Part model, mm, in its own coordinate system. A direction names the side the tool comes from. Coordinates: 2 decimals unless noted, no trailing zeros. Write each loop counter-clockwise with the first axis right and the second up, starting at its lowest first coordinate (ties: lowest second). Pieces come first, ordered by that corner, then holes. Notation, with made-up numbers: (-15, 59.5) - (-4, 59.5) arc R29 cw to (-4, 83.5) - close; hole circle Ø10 at (35, -10.75). An arc over 180 degrees is marked (long way). Use one line per item in the form item = value. Start each with the question number.
from build123d import *

# Parameters (mm, degrees)
SKETCH_1_W          = 367
SKETCH_1_H          = 337
EXTRUDE_1_DEPTH     = 200
SKETCH_2_W          = 245
SKETCH_2_H          = 47
EXTRUDE_2_DEPTH     = 47
SKETCH_3_W          = 18.503948035
SKETCH_3_H          = 22.759447516
EXTRUDE_3_DEPTH     = 35
SKETCH_4_R          = 4.689122638
EXTRUDE_4_DEPTH     = 70
CUT_EXTRUDE_1_DEPTH = 25
CUT_EXTRUDE_2_DEPTH = 223


with BuildPart() as part:
    # Эскиз1 → Бобышка-Вытянуть1 (new body)
    with BuildSketch(Plane(origin=(0, 0, 0), x_dir=(1, 0, 0), z_dir=(0, 1, 0))):
        with Locations((-16.254231815, -121.394753304)):
            Rectangle(SKETCH_1_W, SKETCH_1_H)
    extrude(amount=EXTRUDE_1_DEPTH)

    # Эскиз2 → Бобышка-Вытянуть2 (add)
    with BuildSketch(Plane(origin=(0, 0, -47.105246696), x_dir=(-1, 0, 0), z_dir=(0, 0, -1))):
        with Locations((16.254231815, 23.5)):
            Rectangle(SKETCH_2_W, SKETCH_2_H)
    extrude(amount=EXTRUDE_2_DEPTH)

    # Эскиз3 → Бобышка-Вытянуть3 (add)
    with BuildSketch(Plane(origin=(0, 0, -47.105246696), x_dir=(-1, 0, 0), z_dir=(0, 0, -1))):
        with Locations((-137.993794167, 26.379723758)):
            Rectangle(SKETCH_3_W, SKETCH_3_H)
    extrude(amount=EXTRUDE_3_DEPTH)

    # Эскиз4 → Бобышка-Вытянуть4 (add)
    with BuildSketch(Plane(origin=(0, 0, -82.105246696), x_dir=(-1, 0, 0), z_dir=(0, 0, -1))):
        with Locations((-137.993794168, 26.379723758)):
            Circle(SKETCH_4_R)
    extrude(amount=EXTRUDE_4_DEPTH)

    # Эскиз5 → Вырез-Вытянуть1 (cut)
    with BuildSketch(Plane.XY.offset(289.894753304)):
        with BuildLine():
            Line((-86.254231815, 0), (53.745768185, 0))
            Line((53.745768185, 0), (53.745768185, 17))
            ThreePointArc((53.745768185, 17), (50.816835997, 24.071067812), (43.745768185, 27))
            Line((43.745768185, 27), (-76.254231815, 27))
            ThreePointArc((-76.254231815, 27), (-83.325299626, 24.071067812), (-86.254231815, 17))
            Line((-86.254231815, 17), (-86.254231815, 0))
        make_face()
    extrude(amount=-CUT_EXTRUDE_1_DEPTH, mode=Mode.SUBTRACT)

    # Эскиз6 → Вырез-Вытянуть2 (cut)
    with BuildSketch(Plane(origin=(96.245768185, 0, 0), x_dir=(0, 0, -1), z_dir=(1, 0, 0))):
        with BuildLine():
            Line((-289.894753304, 200), (-56.894753304, 200))
            Line((-56.894753304, 200), (-56.894753304, 140))
            add(Edge.make_bspline(
                [(-289.894753304, 200), (-255.905913973, 199.483070544), (-195.675702754, 150.542684271), (-111.630124679, 134.680175733), (-84.590503935, 135.886366382), (-56.894753304, 140)],
                knots=[0, 0, 0, 0, 0.585078831, 0.685078831, 1, 1, 1, 1], degree=3))
        make_face()
    extrude(amount=-CUT_EXTRUDE_2_DEPTH, mode=Mode.SUBTRACT)


solid = part.part
Q1. Slice it at B-B (y = 90). List the corners of the cut face in (x, z).
Q2. Slice it at A-A (z = -70.5). List the corners of the cut face in (x, y), plus the area to 3 significant figures.
Q3. Mould opens along X. For faces 4 (the cylindrical face through (-83.247, 24.148, 277.57)), 5 (the flat face through (96.246, 175, 146)), 6 (the flat face through (-15, 47, -70)), 7 (the flat face through (-138.754, 23, -70)) say: released by +X, released by -X, zero draft, split by the parting line, or undercut.
Q4. Slice it at C-C (x = -157). List the corners of the cut face in (y, z), plus the area to 3 significant figures.
Q5. Drill centre lines: probe 1 along X at (y, z) = (191.5, 98); probe 2 along Z at (x, y) = (-184.5, 166); probe 3 along Y at (x, z) = (-51.5, -72.5). Where is each one in solid material? Low to high.
Q6. Which spindle directions (+Z, -Z, +X, -X, +Y, -Y) get a long thin tool onto all of the face, cutting with end or side? Do faces 1 (the cylindrical face through (133.52, 27.79, -116.62)), 2 (the flat face through (-17, 14, 264.895)), 3 (the flat face through (-14, 170, 56.895)). Say none if no direction does.
Q7. Pin check, flat tips, straight feed: P1, Ø5.5, axis at x = 138.5, z = -65.5, coming from the +Y side; P2, Ø7, axis at y = 21, z = -59, coming from the +X side; P3, Ø15, axis at x = 135, z = -56.5, coming from the -Y side; P4, Ø15, axis at x = 139.5, y = 31, coming from the -Z side. Stop position of each tip, or through.
Solution:
q1.outline = (-199.75, -47.11) - (167.25, -47.11) - (167.25, 289.89) - (-199.75, 289.89) - close
q2.outline = (-138.75, 0) - (106.25, 0) - (106.25, 47) - (-138.75, 47) - close; (128.74, 15) - (147.25, 15) - (147.25, 37.76) - (128.74, 37.76) - close
q2.area = 11,900 mm2
q3.face_4 = undercut
q3.face_5 = undercut
q3.face_6 = zero draft
q3.face_7 = released by -X
q4.outline = (0, -47.11) - (200, -47.11) - (200, 289.89) - (0, 289.89) - close
q4.area = 67,400 mm2
q5.probe_1 = -199.75 to -126.75, 96.25 to 167.25
q5.probe_2 = -47.11 to 289.89
q5.probe_3 = 0 to 47
q6.face_1 = -Z
q6.face_2 = +Z, -Y
q6.face_3 = +Y
q7.P1 = 37.76
q7.P2 = 147.25
q7.P3 = 15
q7.P4 = -152.11
